For this review, use the dimensioned drawing (mm, ordinates from the lowest corner) and the shaded views. Coordinates: 2 decimals unless noted, no trailing zeros. Loops run counter-clockwise (first coordinate to the right, second up) from the corner with the lowest first, then second, coordinate; pieces in that order, holes last. Notation, with made-up numbers: (-30.75, -24.75) - (22.25, -24.75) arc R30 cw to (22.25, 0.25) - close; hole circle Ø4 at (29, -3). An arc over 180 degrees is marked (long way). Answer in a Markdown table with one row per item. Add a question column.
(1) We need section A-A on y = 0.3. Write out the cut boundary in (x, z), plus the area to 3 significant figures.
(2) We need section B-B on x = 1. Write out the cut boundary in (y, z).
(3) We need section C-C on z = 1. Write out the cut boundary in (x, y).
(4) For line 1 along X through (y, z) = (0.4, 1); line 2 along Z through (x, y) = (7.25, 0.45), list the stretches that pass through material, from the lowest coordinate up.
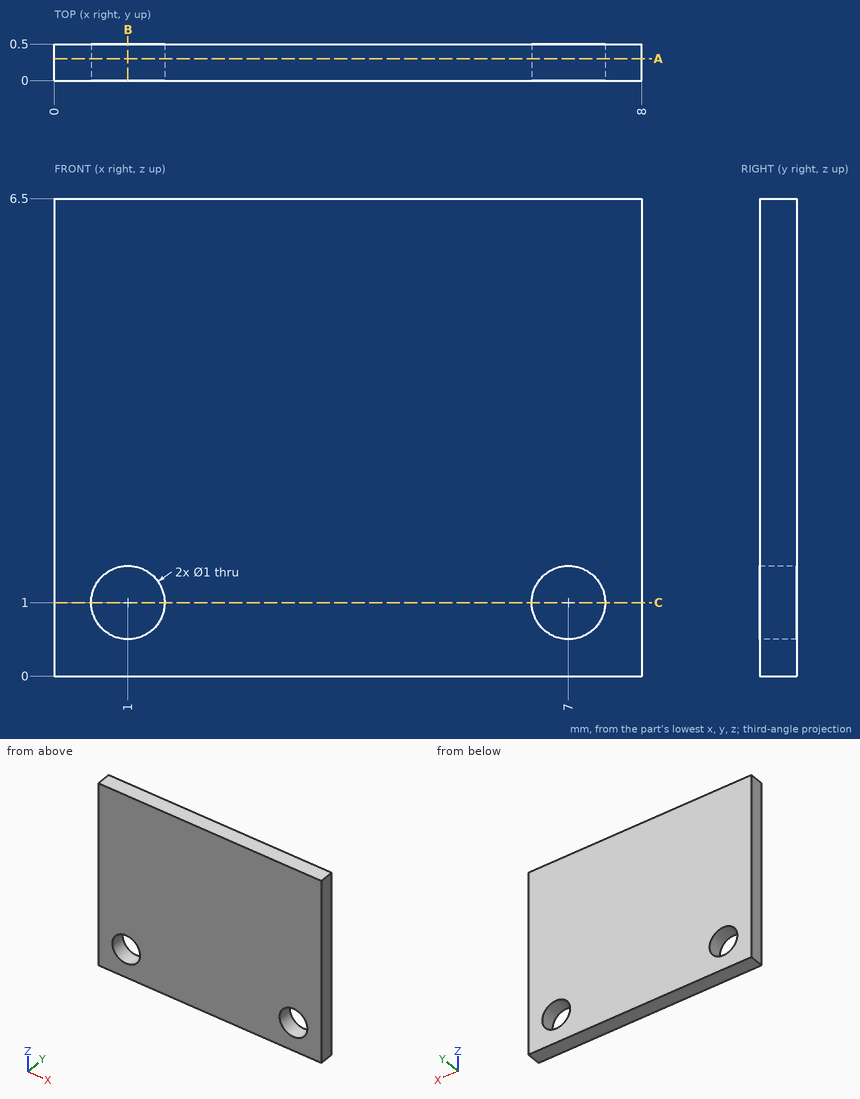
Outcome:
| question | item | result |
|---|---|---|
| 1 | outline | (0, 0) - (8, 0) - (8, 6.5) - (0, 6.5) - close; hole circle Ø1 at (1, 1); hole circle Ø1 at (7, 1) |
| 1 | area | 50.4 mm² |
| 2 | outline | (0, 0) - (0.5, 0) - (0.5, 0.5) - (0, 0.5) - close; (0, 1.5) - (0.5, 1.5) - (0.5, 6.5) - (0, 6.5) - close |
| 3 | outline | (0, 0) - (0.5, 0) - (0.5, 0.5) - (0, 0.5) - close; (1.5, 0) - (6.5, 0) - (6.5, 0.5) - (1.5, 0.5) - close; (7.5, 0) - (8, 0) - (8, 0.5) - (7.5, 0.5) - close |
| 4 | line 1 | 0 to 0.5, 1.5 to 6.5, 7.5 to 8 |
| 4 | line 2 | 0 to 0.57, 1.43 to 6.5 |
